Can you work these out from the drawing? Everything is in mm from the part's minimum corner. Coordinates: 2 decimals unless noted, no trailing zeros. Loops run counter-clockwise (first coordinate to the right, second up) from the corner with the lowest first, then second, coordinate; pieces in that order, holes last. Notation, with made-up numbers: (-19.5, 28.5) - (28.5, 28.5) arc R15 ccw to (28.5, 56.5) - close; hole circle Ø7 at (83, 71). An arc over 180 degrees is marked (long way). One line per question, with ' | ' between items. Start each with the question number.
1. Please list where this line runs through material, in increasing order: L1, parallel to X at y = 16.6, z = 1.2 (3 decimals). Write a range as [from, to].
2. I want a section at B-B, the plane z = 0.95. Count the separate pieces of the cut face and the enclosed holes in it, then the cut area to 3 significant figures.
3. I want a section at A-A, the plane y = 6.04. Write out the boundary of the cut face in (x, z) (3 decimals), then the cut area to 3 significant figures.
4. I want a section at C-C, the plane x = 4. Write out the boundary of the cut face in (y, z) (3 decimals).
5. I'm going to push a flat-ended pin straight in: P1, Ø2, axis at x = 6.5, y = 7, coming from the -Z side. Where does the tip first touch, or does it pass through?
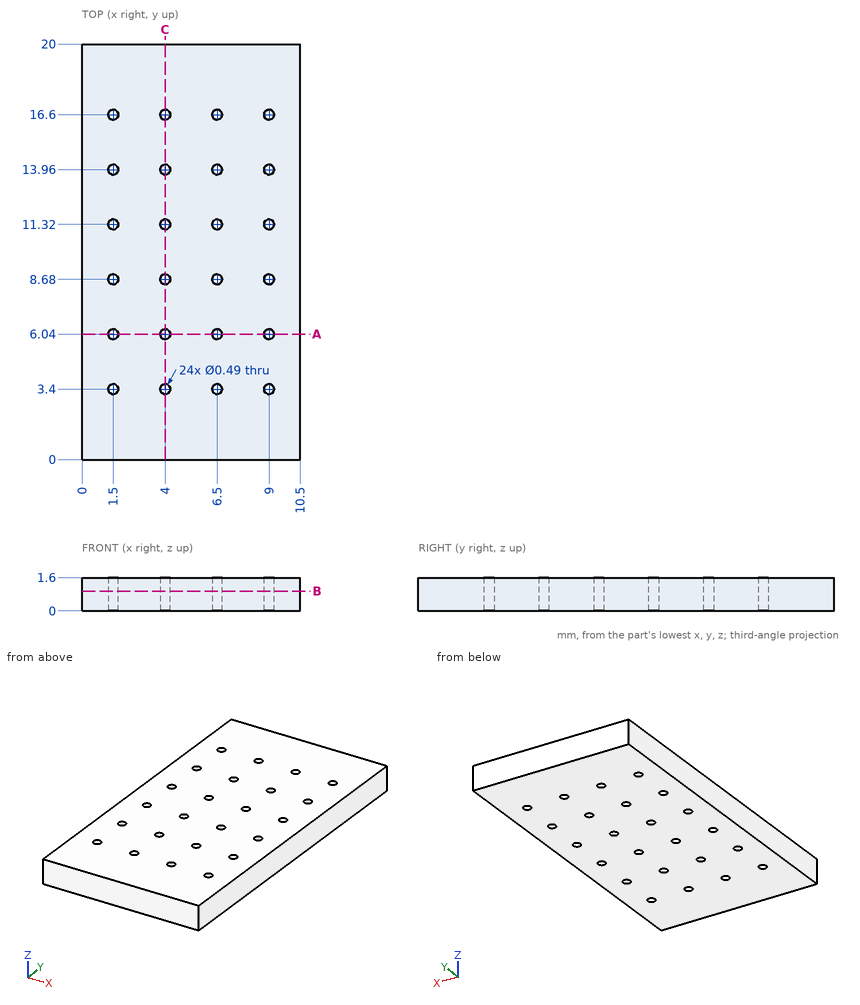
Results are:
1) L1: x = [0, 1.255], [1.745, 3.755], [4.245, 6.255], [6.745, 8.755], [9.245, 10.5]
2) separate pieces: 1 | enclosed holes: 24 | area: 205 mm2
3) outline: (0, 0) - (1.255, 0) - (1.255, 1.6) - (0, 1.6) - close; (1.745, 0) - (3.755, 0) - (3.755, 1.6) - (1.745, 1.6) - close; (4.245, 0) - (6.255, 0) - (6.255, 1.6) - (4.245, 1.6) - close; (6.745, 0) - (8.755, 0) - (8.755, 1.6) - (6.745, 1.6) - close; (9.245, 0) - (10.5, 0) - (10.5, 1.6) - (9.245, 1.6) - close | area: 13.7 mm2
4) outline: (0, 0) - (3.155, 0) - (3.155, 1.6) - (0, 1.6) - close; (3.645, 0) - (5.795, 0) - (5.795, 1.6) - (3.645, 1.6) - close; (6.285, 0) - (8.435, 0) - (8.435, 1.6) - (6.285, 1.6) - close; (8.925, 0) - (11.075, 0) - (11.075, 1.6) - (8.925, 1.6) - close; (11.565, 0) - (13.715, 0) - (13.715, 1.6) - (11.565, 1.6) - close; (14.205, 0) - (16.355, 0) - (16.355, 1.6) - (14.205, 1.6) - close; (16.845, 0) - (20, 0) - (20, 1.6) - (16.845, 1.6) - close
5) P1: stops at z = 0
